Geometry check sheet. Reference: drawing and pictorial views, mm from the part's lowest x, y, z. A direction names the side the tool comes from. Round coordinates to 2 decimals unless told otherwise and drop trailing zeros. Loops run counter-clockwise (first coordinate to the right, second up) from the corner with the lowest first, then second, coordinate; pieces in that order, holes last. Notation, with made-up numbers: (10, 33) -> (59, 33) arc R20 cw to (59, 48) -> close; hole circle Ø8 at (6.5, 28.5). An arc over 180 degrees is marked (long way). Use one line per item in the form item = value.
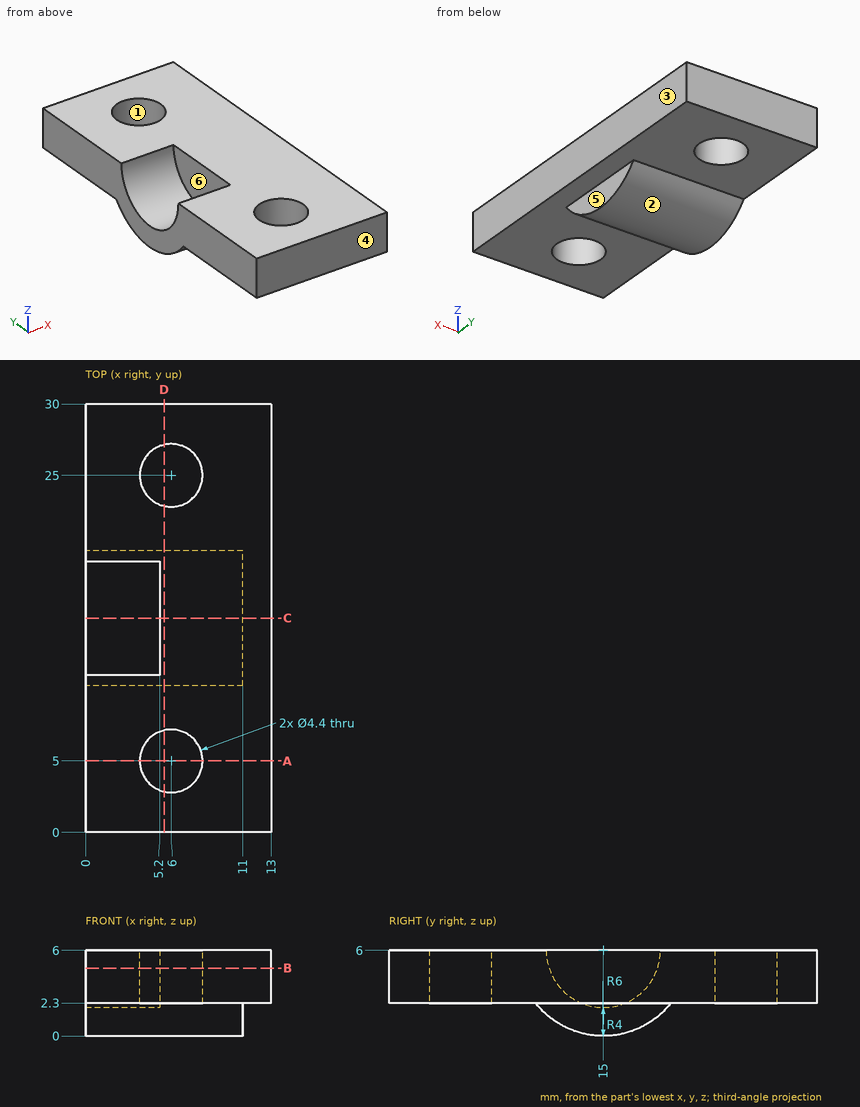
1. Gauge pin test, flat ends, axial feed: pin 1 (5 mm diameter, centred on x = 6, y = 25, fed in from -Z); pin 2 (1.2 mm diameter, centred on y = 16.5, z = 0.5, fed in from +X). Record the tip position at first contact, or that the pin passes through.
Return value:
pin_1 = 2.3
pin_2 = 11
2. Tool access check on the marked faces 4, 5 and 6. Record the directions out of +Z, -Z, +X, -X, +Y, -Y that give a thin tool (end or side, any length) a straight path to the whole face; none if there is none.
Return value:
face_4 = +Z, -Z, +X, -X, -Y
face_5 = -Z, +X, +Y, -Y
face_6 = +Z, -X
3. Mould release check, pull along X, two halves, no side actions. Record for the marked faces 1, 2 and 3: released by +X, released by -X, zero draft, split by the parting line, or undercut.
Return value:
face_1 = undercut
face_2 = zero draft
face_3 = released by +X
4. Section check A-A (y = 5). Record the boundary of the cut face in (x, z), then the cut area to 3 significant figures.
Return value:
outline = (0, 2.3) -> (3.8, 2.3) -> (3.8, 6) -> (0, 6) -> close; (8.2, 2.3) -> (13, 2.3) -> (13, 6) -> (8.2, 6) -> close
area = 31.8 mm2
5. Section check C-C (y = 15). Record the boundary of the cut face in (x, z).
Return value:
outline = (0, 0) -> (11, 0) -> (11, 2.3) -> (13, 2.3) -> (13, 6) -> (5.2, 6) -> (5.2, 2) -> (0, 2) -> close
6. Section check D-D (x = 5.5). Record the boundary of the cut face in (y, z).
Return value:
outline = (0, 2.3) -> (2.86, 2.3) -> (2.86, 6) -> (0, 6) -> close; (7.14, 2.3) -> (10.28, 2.3) arc R6 ccw to (19.72, 2.3) -> (22.86, 2.3) -> (22.86, 6) -> (7.14, 6) -> close; (27.14, 2.3) -> (30, 2.3) -> (30, 6) -> (27.14, 6) -> close
7. Section check B-B (z = 4.75). Record the boundary of the cut face in (x, y).
Return value:
outline = (0, 0) -> (13, 0) -> (13, 30) -> (0, 30) -> (0, 18.8) -> (5.2, 18.8) -> (5.2, 11.2) -> (0, 11.2) -> close; hole circle Ø4.4 at (6, 5); hole circle Ø4.4 at (6, 25)
8. Material ranges on line 1 along Y through (x, z) = (6, 4.05); line 2 along X through (y, z) = (5, 3.5); line 3 along Y through (x, z) = (8, 2.5), recorded low to high.
Return value:
line_1 = 0 to 2.8, 7.2 to 22.8, 27.2 to 30
line_2 = 0 to 3.8, 8.2 to 13
line_3 = 0 to 4.08, 5.92 to 24.08, 25.92 to 30
